Build history of the part. All positions in model axes, mm. A direction names the side the tool comes from. Give positions to 0.01 mm unless a question says otherwise; leave off trailing zeros. Loops run counter-clockwise (first coordinate to the right, second up) from the corner with the lowest first, then second, coordinate; pieces in that order, holes last. Notation, with made-up numbers: M 50,-9 L 55,-9 A22 ccw 55,20 Z; hole C 64,10 d4. An arc over 180 degrees is marked long. Put each result on its own line as item: value.
Autodesk Inventor part; units mm, degrees
ref_plane "YZ Plane" through (0, 0, 0) normal (1, 0, 0) x (0, 1, 0)
ref_plane "XZ Plane" through (0, 0, 0) normal (0, 1, 0) x (-1, 0, 0)
ref_plane "XY Plane" through (0, 0, 0) normal (0, 0, 1) x (1, 0, 0)
sketch "Sketch1" plane through (0, 0, 0) normal (0, 0, 1) x (1, 0, 0)
  line L0 (0, 0) -> (71, 0)
  line L1 (71, 0) -> (71, 42)
  line L2 (71, 42) -> (0, 42)
  line L3 (0, 42) -> (0, 0)
  dimension "d0" = 71
  dimension "d1" = 42
extrude "Extrusion1" add sketch "Sketch1" along normal blind 1.5875
chamfer "Chamfer1" distance 6.35 angle 45 4 edges at (0, 42, 0.7937) (0, 0, 0.7937) (71, 0, 0.7937) (71, 42, 0.7937)
sketch "Sketch2" plane through (0, 0, 1.5875) normal (0, 0, 1) x (1, 0, 0)
  line L0 (0, 6.35) -> (0, 35.65)
  line L1 (71, 35.65) -> (71, 6.35)
  circle A0 centre (3, 21) radius 2
  circle A1 centre (68, 21) radius 2
  line L2 (5, 21) -> (5, 26.1458)
  line L3 (3, 23) -> (0, 23)
  line L4 (3, 19) -> (0, 19)
  line L5 (66, 18.2827) -> (66, 24.0716)
  line L6 (68, 23) -> (71, 23)
  line L7 (68, 19) -> (71, 19)
  line L8 (71, 19) -> (71, 23)
  line L9 (0, 19) -> (0, 23)
  point P0 (0, 0)
  dimension "d7" = 4
  dimension "d8" = 4
  dimension "d10" = 5
  dimension "d11" = 5
extrude "Extrusion2" cut sketch "Sketch2" against normal blind 1.5875
sketch "Sketch3" plane through (0, 0, 1.5875) normal (0, 0, 1) x (1, 0, 0)
  line L0 (71, 19) -> (71, 6.35)
  line L1 (1.5875, 42) -> (69.4125, 42)
  line L2 (69.4125, 42) -> (69.4125, 0)
  line L3 (69.4125, 0) -> (1.5875, 0)
  line L4 (1.5875, 0) -> (1.5875, 42)
  line L5 (0, 40.64) -> (63.5, 40.64)
  line L6 (63.5, 40.64) -> (63.5, 0)
  line L7 (63.5, 0) -> (0, 0)
  line L8 (0, 0) -> (0, 40.64)
  point P0 (0, 0)
  dimension "d14" = 67.825
  dimension "d15" = 1.5875
  dimension "d16" = 63.5
  dimension "d17" = 42
  dimension "d18" = 40.64
properties part number "ElectronicsBoard" material "Phenolic"
Q1. Mould opens along Y. For faces 1 (the flat face through (35, 0, 1)), 2 (the flat face through (0, 29, 1)), 3 (the cylindrical face through (66, 21, 1)) say: pulls with the +Y half, pulls with the -Y half, needs draft (parallel to the pull), parting line crosses it, or undercut.
Here are the results:
face 1: pulls with the -Y half
face 2: needs draft
face 3: undercut
Q2. Slice it at B-B (y = 37). List the corners of the cut face in (x, z), and give its area (3 significant figures).
Here are the results:
outline: M 1.35,0 L 69.65,0 L 69.65,1.59 L 1.35,1.59 Z
area: 108 mm²
Q3. Tool access for faces 4 (the flat face through (67.87, 38.78, 0.78)), 5 (the flat face through (2, 19, 1)), 6 (the flat face through (69, 23, 1)): list every direction of +Z, -Z, +X, -X, +Y, -Y with a clear straight run to the whole face (end or side of a thin tool).
Here are the results:
face 4: +Z, -Z, +X, +Y
face 5: +Z, -Z, -X
face 6: +Z, -Z, +X
Q4. Drop a flat-ended pin along its axis: pin 1 Ø0.8 at (x, z) = (1.5, 0.5) entering from +Y. Give the stop position or say it passes through.
Here are the results:
pin 1: y = 37.55
Q5. Probe line 1 (X direction, y = 36, z = 1.2); line 2 (X direction, y = 5.5, z = 0.15). List the from-to ranges inside material, lowest first. Write a range as from..to.
Here are the results:
line 1: 0.35..70.65
line 2: 0.85..70.15
Q6. Slice it at A-A (z = 0.5). List the corners of the cut face in (x, y).
Here are the results:
outline: M 0,6.35 L 6.35,0 L 64.65,0 L 71,6.35 L 71,19 L 68,19 A2 cw 68,23 L 71,23 L 71,35.65 L 64.65,42 L 6.35,42 L 0,35.65 L 0,23 L 3,23 A2 cw 3,19 L 0,19 Z
